Can you work these out from the model? Positions are in its coordinate system, mm. Give positions to 0.01 mm unless a question says otherwise; leave off trailing zeros. Order: outer loops, then holes, each group sorted by start corner. A loop starts at its lowest first (then second) coordinate and runs counter-clockwise, first axis right, second up. Notation, with made-up numbers: (0, 68) - (41, 68) arc R22 cw to (41, 106) - close; hole circle Ø11 at (43.25, -6.75). An arc over 180 degrees is marked (long way). Answer as a JSON object with one key per item and string values.
```python
from build123d import *

# Parameters (mm, degrees)
ESQUISSE1_W                                    = 4
ESQUISSE1_H                                    = 10.5
CHANFREIN1_SIZE                                = 2.309401077
CHANFREIN1_SIZE_2                              = 4
ENL_V_MAT_EXTRU_2_REACH                        = 39.69
ESQUISSE7_R                                    = 1.7
FRAISAGE_POUR_VIS_T_TE_FRAIS_E_M31_D           = 3.4
FRAISAGE_POUR_VIS_T_TE_FRAIS_E_M31_CSINK_D     = 7.3
FRAISAGE_POUR_VIS_T_TE_FRAIS_E_M31_CSINK_ANGLE = 90
TROU_TARAUD_M31_D                              = 2.5
CHANFREIN2_SIZE                                = 0.5


with BuildPart() as part:
    # Esquisse1 → Révolution1 (revolve)
    with BuildSketch(Plane.XY, mode=Mode.PRIVATE) as r_volution1_sk:
        with Locations((2, 21.25)):
            Rectangle(ESQUISSE1_W, ESQUISSE1_H)
    revolve(r_volution1_sk.sketch.rotate(Axis((0, 0, 0), (1, 0, 0)), 90), axis=Axis((0, 0, 0), (1, 0, 0)))

    # Chanfrein1
    # the kernel refuses this chamfer: 4, 2.309401077 mm, written as the material it takes off along each edge
    with BuildSketch(Plane(origin=(4, 0, 0), x_dir=(0, 0, 1), z_dir=(0, 1, 0))) as chanfrein1_piece_1:
        Polygon((16 + CHANFREIN1_SIZE, 0), (16, -CHANFREIN1_SIZE_2), (16, 0), align=None)
    revolve(axis=Axis((4, 0, 0), (1, 0, 0)), mode=Mode.SUBTRACT)

    # Esquisse7 → Enlèv. mat.-Extru.2 (cut, up to next)
    with BuildSketch(Plane(origin=(4, 0, 0), x_dir=(0, 0, -1), z_dir=(1, 0, 0)), mode=Mode.PRIVATE) as enl_v_mat_extru_2_sk1:
        with Locations((0, -22.5)):
            Circle(ESQUISSE7_R)
    enl_v_mat_extru_2_tool1 = extrude(enl_v_mat_extru_2_sk1.sketch, amount=-ENL_V_MAT_EXTRU_2_REACH, mode=Mode.PRIVATE) & part.part
    add(enl_v_mat_extru_2_tool1.solids().sort_by_distance((4, -22.5, 0))[0], mode=Mode.SUBTRACT)

    # Fraisage pour vis à tête fraisée M31 (through all)
    with Locations(Plane(origin=(4, 0, 0), x_dir=(0, 0, -1), z_dir=(1, 0, 0))):
        with Locations((0, 22.5), (-22.5, 0), (22.5, 0)):
            CounterSinkHole(FRAISAGE_POUR_VIS_T_TE_FRAIS_E_M31_D / 2, FRAISAGE_POUR_VIS_T_TE_FRAIS_E_M31_CSINK_D / 2, counter_sink_angle=FRAISAGE_POUR_VIS_T_TE_FRAIS_E_M31_CSINK_ANGLE)

    # Trou taraudé M31 (through all)
    with Locations(Plane(origin=(4, 0, 0), x_dir=(0, 0, -1), z_dir=(1, 0, 0))):
        with Locations((-15.909902577, -15.909902577)):
            Hole(TROU_TARAUD_M31_D / 2)

    # Chanfrein2
    # the kernel refuses this chamfer: 0.5 mm, written as the material it takes off along each edge
    with BuildSketch(Plane(origin=(4, 0, 0), x_dir=(0, 0, 1), z_dir=(0, 1, 0))) as chanfrein2_piece_1:
        Polygon((26.5, -CHANFREIN2_SIZE), (26.5 - CHANFREIN2_SIZE, 0), (26.5, 0), align=None)
    revolve(axis=Axis((4, 0, 0), (1, 0, 0)), mode=Mode.SUBTRACT)


solid = part.part
```
Q1. We'd pull the mould along Z, two halves only. Please class faces 1 (the face through (2.028, -20.814, 0.221)), 2 (the face through (0, 0, -17)), 3 (the face through (1.774, -26.274, -3.45)): released by +Z, released by -Z, zero draft, split by the parting line, or undercut.
Recorded:
{"face 1": "undercut", "face 2": "zero draft", "face 3": "split by the parting line"}
Q2. I need wall thicknesses on L1, parallel to Y at x = 1.1, z = 0; L2, parallel to Z at x = 2.65, y = 1; L3, parallel to Y at x = 1.3, z = 0. Which ranges of each line are inside material? Lowest first, please.
Recorded:
{"L1": "y = -26.5 to -24.2, -20.8 to -16.64, 16.64 to 20.8, 24.2 to 26.5", "L2": "z = -26.48 to -24.57, -20.43 to -17.5, 17.5 to 20.43, 24.57 to 26.48", "L3": "y = -26.5 to -24.2, -20.8 to -16.75, 16.75 to 20.8, 24.2 to 26.5"}
Q3. If we section it at B-B, the plane z = 0: Please give me the cut outline in (x, y) (3 decimals).
Recorded:
{"outline": "(0, -26.5) - (3.5, -26.5) - (4, -26) - (4, -24.2) - (0, -24.2) - close; (0, -20.8) - (4, -20.8) - (4, -18.309) - (0, -16) - close; (0, 16) - (4, 18.309) - (4, 18.85) - (2.05, 20.8) - (0, 20.8) - close; (0, 24.2) - (2.05, 24.2) - (3.925, 26.075) - (3.5, 26.5) - (0, 26.5) - close"}
Q4. If we section it at A-A, the plane x = 2.75: Please give me the cut outline in (y, z), then the cut area to 3 significant figures.
Recorded:
{"outline": "circle Ø53 at (0, 0); hole circle Ø3.4 at (-22.5, 0); hole circle Ø35.18 at (0, 0); hole circle Ø2.5 at (-15.91, 15.91); hole circle Ø4.8 at (0, -22.5); hole circle Ø4.8 at (0, 22.5); hole circle Ø4.8 at (22.5, 0)", "area": "1,170 mm^2"}
Q5. I'm going to push flat-ended pins straight in: pin 1 Ø1 at (x, y) = (1.5, 20.5) entering from -Z; pin 2 Ø12 at (y, z) = (-15, -0.5) entering from +X; pin 3 Ø2.5 at (y, z) = (22.5, 0) entering from +X; pin 4 Ø1 at (x, y) = (3.5, -7.5) entering from +Z. Where does each tip first touch, or does it pass through?
Recorded:
{"pin 1": "stops at z = -17.39", "pin 2": "stops at x = 4", "pin 3": "passes through", "pin 4": "stops at z = 25.56"}
